Read the model definition and answer for the solid it produces. Units are mm, in the model's axes. A direction names the side the tool comes from. Coordinates: 2 decimals unless noted, no trailing zeros. Loops run counter-clockwise (first coordinate to the right, second up) from the corner with the lowest first, then second, coordinate; pieces in that order, holes last. Notation, with made-up numbers: M 86.5,-29 L 99.5,-29 A24 ccw 99.5,-19 Z; hole C 84,16 d6. An arc over 180 degrees is marked long. Put each result on its own line as item: value.
from build123d import *

# Parameters (mm, degrees)
SKETCH1_W               = 70
SKETCH1_H               = 70
BOSS_EXTRUDE1_DEPTH     = 52.45
CUT_EXTRUDE2_DEPTH      = 95.212538974
CUT_EXTRUDE2_DEPTH_BACK = 70
SKETCH2_W               = 60
SKETCH2_H               = 47.45
SKETCH3_W               = 10
SKETCH3_H               = 10
SKETCH3_R               = 2
BOSS_EXTRUDE2_DEPTH     = 5
SKETCH4_R               = 3.175
CUT_EXTRUDE3_DEPTH      = 5
SKETCH5_W               = 50
SKETCH5_H               = 47.45
CUT_EXTRUDE4_DEPTH      = 80


with BuildPart() as part:
    # Sketch1 → Boss-Extrude1 (new body)
    with BuildSketch(Plane(origin=(0, 0, 0), x_dir=(1, 0, 0), z_dir=(0, 1, 0))):
        Rectangle(SKETCH1_W, SKETCH1_H)
    extrude(amount=BOSS_EXTRUDE1_DEPTH)

    # Sketch2 → Cut-Extrude2 (cut, two sides: drawn at the far end of the back side and taken through both)
    with BuildSketch(Plane.XY.offset(35).offset(-CUT_EXTRUDE2_DEPTH_BACK)):
        with Locations((0, 23.725)):
            Rectangle(SKETCH2_W, SKETCH2_H)
    extrude(amount=CUT_EXTRUDE2_DEPTH + CUT_EXTRUDE2_DEPTH_BACK, mode=Mode.SUBTRACT)

    # Sketch3 → Boss-Extrude2 (add)
    # profile 1 of 4: a face of its own
    with BuildSketch(Plane(origin=(0, 0, 0), x_dir=(1, 0, 0), z_dir=(0, 1, 0))):
        with Locations((40, -30)):
            Rectangle(SKETCH3_W, SKETCH3_H)
        with Locations(Location((40, -30, 0), (0, 0, 270))):
            Circle(SKETCH3_R, mode=Mode.SUBTRACT)
    # profile 2 of 4: a face of its own
    with BuildSketch(Plane(origin=(0, 0, 0), x_dir=(1, 0, 0), z_dir=(0, 1, 0))):
        with Locations((40, 30)):
            Rectangle(SKETCH3_W, SKETCH3_H)
        with Locations(Location((40, 30, 0), (0, 0, 90))):
            Circle(SKETCH3_R, mode=Mode.SUBTRACT)
    # profile 3 of 4: a face of its own
    with BuildSketch(Plane(origin=(0, 0, 0), x_dir=(1, 0, 0), z_dir=(0, 1, 0))):
        with Locations((-40, -30)):
            Rectangle(SKETCH3_W, SKETCH3_H)
        with Locations(Location((-40, -30, 0), (0, 0, 90))):
            Circle(SKETCH3_R, mode=Mode.SUBTRACT)
    # profile 4 of 4: a face of its own
    with BuildSketch(Plane(origin=(0, 0, 0), x_dir=(1, 0, 0), z_dir=(0, 1, 0))):
        with Locations((-40, 30)):
            Rectangle(SKETCH3_W, SKETCH3_H)
        with Locations(Location((-40, 30, 0), (0, 0, 270))):
            Circle(SKETCH3_R, mode=Mode.SUBTRACT)
    extrude(amount=BOSS_EXTRUDE2_DEPTH)

    # Sketch4 → Cut-Extrude3 (cut)
    with BuildSketch(Plane(origin=(0, 52.45, 0), x_dir=(1, 0, 0), z_dir=(0, 1, 0))):
        with Locations(Location((0, 0, 0), (0, 0, 270))):
            Circle(SKETCH4_R)
    extrude(amount=-CUT_EXTRUDE3_DEPTH, mode=Mode.SUBTRACT)

    # Sketch5 → Cut-Extrude4 (cut)
    with BuildSketch(Plane(origin=(35, 0, 0), x_dir=(0, 0, -1), z_dir=(1, 0, 0))):
        with Locations((0, 23.725)):
            Rectangle(SKETCH5_W, SKETCH5_H)
    extrude(amount=-CUT_EXTRUDE4_DEPTH, mode=Mode.SUBTRACT)


solid = part.part
1) Which of the six approach directions +Z, -Z, +X, -X, +Y, -Y give full straight-line access (tool end or side, diameter ignored) to faces 1 (the flat face through (-45, 2, 30)), 2 (the flat face through (30, 23, 30)), 3 (the flat face through (-35, 48, 0)), 4 (the flat face through (37, 0, 30)), 5 (the flat face through (-34, 18, 25))?
Answer list:
face 1: +Z, -Z, -X, +Y, -Y
face 2: +Z, -Z, -Y
face 3: +Z, -Z, -X, +Y
face 4: +Z, -Z, +X, -X, -Y
face 5: +X, -X, -Y
2) Find section C-C, the plane x = 40. Write down the section's boundary in (y, z), plus the area to 3 significant figures.
Answer list:
outline: M 0,-35 L 5,-35 L 5,-32 L 0,-32 Z; M 0,-28 L 5,-28 L 5,-25 L 0,-25 Z; M 0,25 L 5,25 L 5,28 L 0,28 Z; M 0,32 L 5,32 L 5,35 L 0,35 Z
area: 60.0 mm^2
3) Straight lines are drawn through the part: line 1 (X direction, y = 3.15, z = -30); line 2 (X direction, y = 49, z = 0) (3 decimals); line 3 (X direction, y = 37, z = 26). For each, find the intervals that lie inside material, in ascending order. Write a range as [from, to].
Answer list:
line 1: x = [-45, -42], [-38, -30], [30, 38], [42, 45]
line 2: x = [-35, -3.175], [3.175, 35]
line 3: x = [-35, -30], [30, 35]
4) Determine the mould class of faces 6 (the cylindrical face through (38.226, 2.465, 30.923)), 7 (the flat face through (-4, 49, 35)), 8 (the flat face through (-37.8, 5, 29.9)) for opening direction Z: released by +Z, released by -Z, zero draft, split by the parting line, or undercut.
Answer list:
face 6: undercut
face 7: released by +Z
face 8: zero draft
5) Given pin 1 Ø10 at (y, z) = (8, 25) entering from -X; pin 2 Ø8 at (x, z) = (-40.5, -29.5) entering from +Y; pin 3 Ø21 at (x, z) = (2, -8.5) entering from -Y; pin 4 Ø5 at (y, z) = (41, 25) entering from +X, each flat-ended and moving along its own axis, determine where each tip first touches the part or whether it passes through.
Answer list:
pin 1: stops at x = -45
pin 2: stops at y = 5
pin 3: stops at y = 47.45
pin 4: stops at x = 35
6) Find section B-B, the plane y = 21. Write down the section's boundary in (x, z), plus the area to 3 significant figures.
Answer list:
outline: M -35,-35 L -30,-35 L -30,-25 L -35,-25 Z; M -35,25 L -30,25 L -30,35 L -35,35 Z; M 30,-35 L 35,-35 L 35,-25 L 30,-25 Z; M 30,25 L 35,25 L 35,35 L 30,35 Z
area: 200 mm^2
7) Find section D-D, the plane x = 0. Write down the section's boundary in (y, z) (3 decimals), plus the area to 3 significant figures.
Answer list:
outline: M 47.45,-35 L 52.45,-35 L 52.45,-3.175 L 47.45,-3.175 Z; M 47.45,3.175 L 52.45,3.175 L 52.45,35 L 47.45,35 Z
area: 318 mm^2
8) Find section A-A, the plane z = 30. Write down the section's boundary in (x, y).
Answer list:
outline: M -45,0 L -42,0 L -42,5 L -45,5 Z; M -38,0 L -30,0 L -30,47.45 L 30,47.45 L 30,0 L 38,0 L 38,5 L 35,5 L 35,52.45 L -35,52.45 L -35,5 L -38,5 Z; M 42,0 L 45,0 L 45,5 L 42,5 Z
